Read the model definition and answer for the solid it produces. Units are mm, in the model's axes. A direction names the side the tool comes from. Coordinates: 2 decimals unless noted, no trailing zeros. Loops run counter-clockwise (first coordinate to the right, second up) from the corner with the lowest first, then second, coordinate; pieces in that order, holes last.
Autodesk Inventor part; units mm, degrees
ref_plane "YZ Plane" through (0, 0, 0) normal (1, 0, 0) x (0, 1, 0)
ref_plane "XZ Plane" through (0, 0, 0) normal (0, 1, 0) x (-1, 0, 0)
ref_plane "XY Plane" through (0, 0, 0) normal (0, 0, 1) x (1, 0, 0)
sketch "Sketch1" plane through (0, 0, 0) normal (0, 1, 0) x (-1, 0, 0)
  line L0 (198.4375, -231.775) -> (-198.4375, -231.775)
  line L1 (-198.4375, -231.775) -> (-198.4375, 231.775)
  line L2 (-198.4375, 231.775) -> (198.4375, 231.775)
  line L3 (198.4375, 231.775) -> (198.4375, -231.775)
  line L4 (0, -324.485) -> (0, 324.485)
  line L5 (277.8125, 0) -> (-277.8125, 0)
  point P0 (0, 0)
  dimension "d0" = 396.875
  dimension "d1" = 463.55
  dimension "d4" = 198.4375
  dimension "d8" = 231.775
extrude "Shelf Board" add sketch "Sketch1" along normal blind 19.05
sketch "Sketch3" plane through (0, 0, 0) normal (0, -1, 0) x (1, 0, 0)
  line L0 (-198.4375, 231.775) -> (198.4375, 231.775)
  line L1 (-128.5875, 231.775) -> (-90.4875, 231.775)
  line L2 (-90.4875, 231.775) -> (-90.4875, -180.975)
  line L3 (-90.4875, -180.975) -> (-128.5875, -180.975)
  line L4 (-128.5875, -180.975) -> (-128.5875, 231.775)
  line L5 (-198.4375, -231.775) -> (198.4375, -231.775)
  line L6 (-198.4375, 231.775) -> (-198.4375, -231.775)
  line L7 (-14.2875, 231.775) -> (23.8125, 231.775)
  line L8 (23.8125, 231.775) -> (23.8125, -180.975)
  line L9 (23.8125, -180.975) -> (-14.2875, -180.975)
  line L10 (-14.2875, -180.975) -> (-14.2875, 231.775)
  line L11 (198.4375, 231.775) -> (-198.4375, 231.775)
  line L12 (100.0125, 231.775) -> (138.1125, 231.775)
  line L13 (138.1125, 231.775) -> (138.1125, -180.975)
  line L14 (138.1125, -180.975) -> (100.0125, -180.975)
  line L15 (100.0125, -180.975) -> (100.0125, 231.775)
  line L16 (198.4375, 231.775) -> (198.4375, -231.775)
  line L17 (-198.4375, 231.775) -> (198.4375, 231.775)
  line L18 (198.4375, 231.775) -> (198.4375, 219.075)
  line L19 (198.4375, 219.075) -> (-198.4375, 219.075)
  line L20 (-198.4375, 219.075) -> (-198.4375, 231.775)
  point P0 (0, 0)
  dimension "d11" = 50.8
  dimension "d12" = 38.1
  dimension "d13" = 69.85
  dimension "d20" = 12.7
  dimension "d22" = 396.875
  dimension "d25" = 76.2
  dimension "d26" = 76.2
  dimension "d27" = 60.325
extrude "Light Stop Dados" cut sketch "Sketch3" against normal blind 9.525 contours L0 L4 L19 L6 | L0 L2 L19 L4 | L0 L10 L19 L2 | L19 L2 L3 L4 | L0 L8 L19 L10 | L0 L15 L19 L8 | L19 L8 L9 L10 | L19 L13 L0 L16 | L0 L13 L19 L15 | L13 L14 L15 L19
equation "\"d4\" = 0.5 * d0"
equation "\"d8\" = 0.5 * d1"
properties part number "Horizontal Shelf with Lights Left"
Q1. Flat-ended cylindrical pins translate along their axes: pin 1 Ø5 at (x, y) = (-168.5, 3.5) entering from +Z (3 decimals); pin 2 Ø3 at (x, y) = (132, 3.5) entering from +Z (3 decimals). Find the tip coordinate at first contact, or state that the pin passes through.
Findings below:
pin 1: stops at z = 219.075
pin 2: stops at z = -180.975
Q2. Straight lines are drawn through the part: probe 1 along X at (y, z) = (3.75, 90); probe 2 along Y at (x, z) = (129, 93) (3 decimals); probe 3 along Z at (x, y) = (32, 8) (3 decimals). For each, find the intervals that lie inside material, in ascending order.
Findings below:
probe 1: x = -198.44 to -128.59, -90.49 to -14.29, 23.81 to 100.01, 138.11 to 198.44
probe 2: y = 9.525 to 19.05
probe 3: z = -231.775 to 219.075
Q3. Which of the six approach directions +Z, -Z, +X, -X, +Y, -Y give full straight-line access (tool end or side, diameter ignored) to faces 1 (the face through (169, 5, 219.075)), 2 (the face through (-90.488, 5, 22)), 3 (the face through (198.438, 9, -3))?
Findings below:
face 1: +Z, +X, -X, -Y
face 2: +Z, -Y
face 3: +Z, -Z, +X, +Y, -Y
Q4. A cutting plane is placed at C-C (x = 126). Give the vertices of the cut face in (y, z) (3 decimals).
Findings below:
outline: (0, -231.775) - (19.05, -231.775) - (19.05, 231.775) - (9.525, 231.775) - (9.525, -180.975) - (0, -180.975) - close
Q5. A cutting plane is placed at B-B (y = 3.25). Give the vertices of the cut face in (x, z) (1 decimal).
Findings below:
outline: (-198.4, -231.8) - (198.4, -231.8) - (198.4, 219.1) - (138.1, 219.1) - (138.1, -181) - (100, -181) - (100, 219.1) - (23.8, 219.1) - (23.8, -181) - (-14.3, -181) - (-14.3, 219.1) - (-90.5, 219.1) - (-90.5, -181) - (-128.6, -181) - (-128.6, 219.1) - (-198.4, 219.1) - close
